Read the model definition and answer for the solid it produces. Units are mm, in the model's axes. A direction names the side the tool comes from. Coordinates: 2 decimals unless noted, no trailing zeros. Write each loop counter-clockwise with the first axis right and the second up, starting at its lowest first coordinate (ties: lowest second). Pieces come first, ordered by that corner, then holes.
Item 1: Determine the mould class of faces 4 (the face through (-8, 16.169, 0)), 5 (the face through (-7.808, -16.984, 1.494)), 6 (the face through (-7.808, 16.984, -1.494)), 7 (the face through (-8, -16.169, 0)) for opening direction Z: released by +Z, released by -Z, zero draft, split by the parting line, or undercut.
Item 2: Straight lines are drawn through the part: probe 1 along Y at (x, z) = (1.5, 0); probe 2 along X at (y, z) = (-13, -3); probe 3 along Z at (x, y) = (-2.5, 15.5). For each, find the intervals that lie inside material, in ascending order.
Item 3: A tool of negligible diameter and unlimited length cuts with its end or side. For faces 1 (the face through (0, -8, 8)), 2 (the face through (-7.81, -15.92, 2.82)), 3 (the face through (-7.808, 15.925, 2.8)), from which of +Z, -Z, +X, -X, +Y, -Y can it reach the whole face along a straight path? Write none if from no direction.
Item 4: Section A-A (y = 0) is taken. Give the vertices of the cut face in (x, z), then the cut area to 3 significant figures.
Item 5: Each of these flat-tipped pins is pushed along its axis until it touches: P1, Ø6, axis at x = -11.5, z = -6.5, coming from the +Y side; P2, Ø13.5, axis at y = 0, z = 0, coming from the +X side; P3, Ø10, axis at y = -1, z = -4.5, coming from the +X side; P4, Ø5, axis at x = -13.5, z = -13, coming from the +Y side. Where does it stop, or does it pass through?
Item 6: Section C-C (x = 4.5) is taken. Give the vertices of the cut face in (y, z).
from build123d import *

# Parameters (mm, degrees)
EXTRUSION1_DEPTH             = 45.079643828
R_P_TITION_CIRCULAIRE1_COUNT = 36


with BuildPart() as part:
    # Esquisse1 → Révolution1 (revolve)
    with BuildSketch(Plane.XY, mode=Mode.PRIVATE) as r_volution1_sk:
        Polygon((21.5, 8.5), (21.5, 11), (0, 11), (0, 17.05), (-15.4, 17.05), (-15.4, 11), (-25.4, 11), (-25.4, 8.5), (-3.228913747, 8.5), (-3.228913747, 7.497868496), (16.5, 7.497868496), (16.5, 8.5), align=None)
    revolve(r_volution1_sk.sketch.rotate(Axis((-31.537627468, 0, 0), (1, 0, 0)), 90), axis=Axis((-31.537627468, 0, 0), (1, 0, 0)))

    # Esquisse2 → Extrusion1 (cut, through all)
    with BuildSketch(Plane.ZY.offset(15.4)):
        Polygon((-1, 17.131935336), (-0.551103456, 16.169273591), (0.551103456, 16.169273591), (1, 17.131935336), align=None)
    extrusion1 = extrude(amount=-EXTRUSION1_DEPTH, mode=Mode.SUBTRACT)

    # Répétition circulaire1: Extrusion1 ×36 about axis
    r_p_tition_circulaire1_axis = Axis((0, 0, 0), (1, 0, 0))
    for i in range(1, R_P_TITION_CIRCULAIRE1_COUNT):
        add(extrusion1.rotate(r_p_tition_circulaire1_axis, i * 360 / R_P_TITION_CIRCULAIRE1_COUNT), mode=Mode.SUBTRACT)


solid = part.part
Established:
1. face 4: undercut
1. face 5: released by +Z
1. face 6: released by -Z
1. face 7: undercut
2. probe 1: y = -11 to -7.5, 7.5 to 11
2. probe 2: x = -15.4 to 0
2. probe 3: z = -7.1 to -6.54, -5 to 5, 6.54 to 7.1
3. face 1: +X
3. face 2: +X, -X, -Y
3. face 3: +X, -X, +Y
4. outline: (-25.4, -11) - (-15.4, -11) - (-15.4, -16.17) - (0, -16.17) - (0, -11) - (21.5, -11) - (21.5, -8.5) - (16.5, -8.5) - (16.5, -7.5) - (-3.23, -7.5) - (-3.23, -8.5) - (-25.4, -8.5) - close; (-25.4, 8.5) - (-3.23, 8.5) - (-3.23, 7.5) - (16.5, 7.5) - (16.5, 8.5) - (21.5, 8.5) - (21.5, 11) - (0, 11) - (0, 16.17) - (-15.4, 16.17) - (-15.4, 11) - (-25.4, 11) - close
4. area: 433 mm2
5. P1: stops at y = 16.6
5. P2: passes through
5. P3: stops at x = 21.5
5. P4: stops at y = 12.43
6. outline: circle Ø22 at (0, 0); hole circle Ø15 at (0, 0)
